Part model, mm, in its own coordinate system. Face numbers are marked on the shaded views. A direction names the side the tool comes from. Give positions to 0.01 mm unless a question says otherwise; leave off trailing zeros. Order: outer loops, then holes, each group sorted by start corner. A loop starts at its lowest first (then second) coordinate and runs counter-clockwise, first axis right, second up. Notation, with made-up numbers: M 72.5,38 L 122.5,38 A7 cw 122.5,51 Z; hole C 7.25,-38 d3. An arc over 180 degrees is marked long. One line per question, with ' | ' between items.
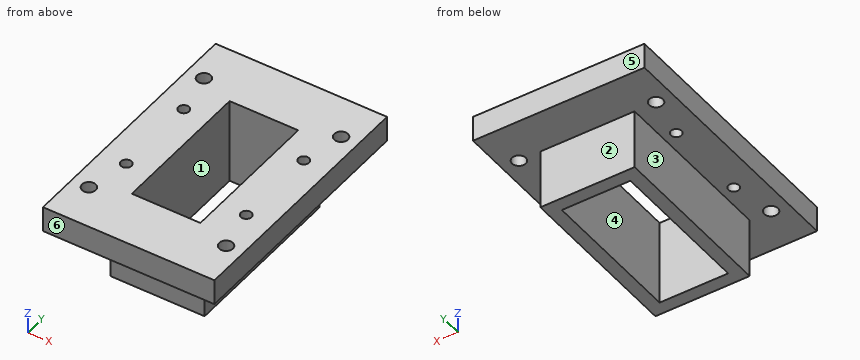
```python
from build123d import *

# Parameters (mm, degrees)
SKETCH1_W               = 40
SKETCH1_H               = 60
BOSS_EXTRUDE1_DEPTH     = 6
M3_CLEARANCE_HOLE1_D    = 3.2
CUT_EXTRUDE1_DEPTH      = 73.360210061
CUT_EXTRUDE1_DEPTH_BACK = 73.360210061
SKETCH4_W               = 22
SKETCH4_H               = 40
SKETCH6_W               = 22
SKETCH6_H               = 40
SKETCH6_W_2             = 16
SKETCH6_H_2             = 34
BOSS_EXTRUDE2_DEPTH     = 20
TAP_DRILL_FOR_M3_TAP2_D = 2.5


with BuildPart() as part:
    # Sketch1 → Boss-Extrude1 (new body)
    with BuildSketch(Plane.XY):
        with Locations((20, 30)):
            Rectangle(SKETCH1_W, SKETCH1_H)
    extrude(amount=BOSS_EXTRUDE1_DEPTH)

    # M3 Clearance Hole1 (through all)
    with Locations(Plane.XY.offset(6)):
        with Locations((4, 10), (4, 50), (36, 50), (36, 10)):
            Hole(M3_CLEARANCE_HOLE1_D / 2)

    # Sketch4 → Cut-Extrude1 (cut, two sides: drawn at the far end of the back side and taken through both)
    with BuildSketch(Plane.XY.offset(6).offset(-CUT_EXTRUDE1_DEPTH_BACK)):
        with Locations((20, 30)):
            Rectangle(SKETCH4_W, SKETCH4_H)
    extrude(amount=CUT_EXTRUDE1_DEPTH + CUT_EXTRUDE1_DEPTH_BACK, mode=Mode.SUBTRACT)

    # Sketch6 → Boss-Extrude2 (add)
    with BuildSketch(Plane(origin=(0, 0, 6), x_dir=(-1, 0, 0), z_dir=(0, 0, -1))):
        with Locations((-20, 30)):
            Rectangle(SKETCH6_W, SKETCH6_H)
        with Locations((-20, 30)):
            Rectangle(SKETCH6_W_2, SKETCH6_H_2, mode=Mode.SUBTRACT)
    extrude(amount=BOSS_EXTRUDE2_DEPTH)

    # Tap Drill for M3 Tap2 (through all)
    with Locations(Plane.XY.offset(6)):
        with Locations((34, 40), (6, 40), (6, 20), (34, 20)):
            Hole(TAP_DRILL_FOR_M3_TAP2_D / 2)


solid = part.part
```
1. Tool access for the marked faces 1, 2 and 3: list every direction of +Z, -Z, +X, -X, +Y, -Y with a clear straight run to the whole face (end or side of a thin tool).
Worked out:
face 1: +Z, -Z | face 2: -Z, +X, -X, +Y | face 3: -Z, -X, +Y, -Y
2. Drop flat-ended pins along their axis: pin 1 (4 mm diameter, centred on x = 9.5, z = -3, fed in from -Y); pin 2 (3 mm diameter, centred on x = 6, y = 40, fed in from -Z); pin 3 (2 mm diameter, centred on x = 6, y = 20, fed in from +Z); pin 4 (11 mm diameter, centred on x = 22.5, z = -10.5, fed in from +Y). Give the stop position or say it passes through.
Worked out:
pin 1: stops at y = 10 | pin 2: stops at z = 0 | pin 3: passes through | pin 4: stops at y = 50
3. Slice it at A-A on x = 36. Give the cut face in (y, z), then the cut area to 3 significant figures.
Worked out:
outline: M 0,0 L 8.4,0 L 8.4,6 L 0,6 Z; M 11.6,0 L 48.4,0 L 48.4,6 L 11.6,6 Z; M 51.6,0 L 60,0 L 60,6 L 51.6,6 Z | area: 322 mm2
4. Slice it at D-D on z = -3.5. Give the cut face in (x, y).
Worked out:
outline: M 9,10 L 31,10 L 31,50 L 9,50 Z; hole M 12,13 L 28,13 L 28,47 L 12,47 Z
5. Mould opens along Y. For the marked faces 4, 5 and 6 say: released by +Y, released by -Y, zero draft, split by the parting line, or undercut.
Worked out:
face 4: undercut | face 5: released by +Y | face 6: released by -Y
6. Slice it at C-C on x = 27. Give the cut face in (y, z), then the cut area to 3 significant figures.
Worked out:
outline: M 0,0 L 10,0 L 10,-14 L 13,-14 L 13,6 L 0,6 Z; M 47,-14 L 50,-14 L 50,0 L 60,0 L 60,6 L 47,6 Z | area: 240 mm2
7. Probe L1, parallel to Y at x = 6, z = 3.8; L2, parallel to Y at x = 4, z = 3.5; L3, parallel to Y at x = 27.5, z = -4.5. List the from-to ranges inside material, lowest first. Write a range as from..to.
Worked out:
L1: y = 0..18.75, 21.25..38.75, 41.25..60 | L2: y = 0..8.4, 11.6..48.4, 51.6..60 | L3: y = 10..13, 47..50
8. Slice it at B-B on y = 37.5. Give the cut face in (x, z).
Worked out:
outline: M 0,0 L 9,0 L 9,-14 L 12,-14 L 12,6 L 0,6 Z; M 28,-14 L 31,-14 L 31,0 L 40,0 L 40,6 L 28,6 Z
